Geometry: final body of the model. Coordinates: model frame, mm. A direction names the side the tool comes from. Round coordinates to 2 decimals unless told otherwise and drop trailing zeros. Order: outer loops, then holes, each group sorted by start corner. A loop starts at its lowest first (then second) coordinate and runs counter-clockwise, first axis right, second up. Notation, with made-up numbers: (-30.75, 47.5) -> (-2.75, 47.5) arc R21 cw to (-2.75, 86.5) -> close; hole circle Ø2 at (-6, 42.25). An arc over 180 degrees is marked (long way). Put each result on its own line as item: value.
```python
from build123d import *

# Parameters (mm, degrees)
CROQUIS1_R              = 2.175
SALIENTE_EXTRUIR1_DEPTH = 2
CROQUIS2_W              = 50
CROQUIS2_H              = 25
CORTAR_EXTRUIR1_DEPTH   = 2
REDONDEO1_R             = 5
CORTAR_EXTRUIR2_DEPTH   = 2


with BuildPart() as part:
    # Croquis1 → Saliente-Extruir1 (new body)
    with BuildSketch(Plane(origin=(0, 0, 0), x_dir=(1, 0, 0), z_dir=(0, 1, 0))):
        with BuildLine():
            Line((-59.24665691, 17.931526281), (-59.24665691, -17.931526281))
            ThreePointArc((-59.24665691, -17.931526281), (-56.317724722, -25.002594093), (-49.24665691, -27.931526281))
            Line((-49.24665691, -27.931526281), (-31.500611182, -27.931526281))
            Line((-31.500611182, -27.931526281), (37.914147183, -27.931526281))
            Line((37.914147183, -27.931526281), (59.24665691, -27.931526281))
            Line((59.24665691, -27.931526281), (59.24665691, 17.931526281))
            ThreePointArc((59.24665691, 17.931526281), (56.317724722, 25.002594093), (49.24665691, 27.931526281))
            Line((49.24665691, 27.931526281), (-49.24665691, 27.931526281))
            ThreePointArc((-49.24665691, 27.931526281), (-56.317724722, 25.002594093), (-59.24665691, 17.931526281))
        make_face()
        with Locations((51.3850757, -20.916819625)):
            Circle(CROQUIS1_R, mode=Mode.SUBTRACT)
        with Locations((-41.6149243, -20.916819625)):
            Circle(CROQUIS1_R, mode=Mode.SUBTRACT)
        with Locations((-41.6149243, 20.083180375)):
            Circle(CROQUIS1_R, mode=Mode.SUBTRACT)
        with Locations((51.3850757, 20.083180375)):
            Circle(CROQUIS1_R, mode=Mode.SUBTRACT)
    extrude(amount=SALIENTE_EXTRUIR1_DEPTH)

    # Croquis2 → Cortar-Extruir1 (cut)
    with BuildSketch(Plane(origin=(0, 2, 0), x_dir=(1, 0, 0), z_dir=(0, 1, 0))):
        with Locations((16.3850757, 15.431526281)):
            Rectangle(CROQUIS2_W, CROQUIS2_H)
    extrude(amount=-CORTAR_EXTRUIR1_DEPTH, mode=Mode.SUBTRACT)

    # Redondeo1
    redondeo1_edges = [part.edges().sort_by_distance(p)[0] for p in [
        (41.3850757, 1, -2.931526281),
        (-8.6149243, 1, -2.931526281),
    ]]
    fillet(redondeo1_edges, radius=REDONDEO1_R)

    # Croquis4 → Cortar-Extruir2 (cut)
    with BuildSketch(Plane.XZ):
        with BuildLine():
            Line((29.444521437, 1.568473719), (30.11759836, 1.568473719))
            Line((30.11759836, 1.568473719), (30.11759836, 4.060260578))
            add(Edge.make_bspline(
                [(30.11759836, 4.060260578), (30.148105822, 4.029289813), (30.208706879, 3.967768435), (30.305496315, 3.881954316), (30.405978505, 3.802124559), (30.511147814, 3.729037402), (30.61962941, 3.661651481), (30.732531913, 3.600498497), (30.849036967, 3.544732313), (30.929745062, 3.513567679), (30.970162463, 3.497960898)],
                knots=[0, 0, 0, 0, 0.000130388, 0.000259007, 0.000387777, 0.000515175, 0.000643004, 0.000770695, 0.000900222, 0.001030157, 0.001030157, 0.001030157, 0.001030157], degree=3))
            Line((30.970162463, 3.497960898), (30.970162463, 4.171037821))
            add(Edge.make_bspline(
                [(30.970162463, 4.171037821), (30.925337531, 4.187845247), (30.831522436, 4.223021882), (30.693082905, 4.297844367), (30.548583301, 4.390482153), (30.427195385, 4.481338367), (30.33081837, 4.562116803), (30.263458163, 4.62704999), (30.201045059, 4.693544942), (30.145925041, 4.763747872), (30.096651183, 4.836239432), (30.052992396, 4.910901194), (30.014562629, 4.987969009), (29.994444914, 5.041637327), (29.984385219, 5.068473719)],
                knots=[0, 0, 0, 0, 0.000143475, 0.000300282, 0.000470852, 0.000658192, 0.000754698, 0.000847923, 0.000938715, 0.001028066, 0.00111538, 0.001201478, 0.001287394, 0.001373323, 0.001373323, 0.001373323, 0.001373323], degree=3))
            Line((29.984385219, 5.068473719), (29.444521437, 5.068473719))
            Line((29.444521437, 5.068473719), (29.444521437, 1.568473719))
        make_face()
        with BuildLine():
            Line((0.238227731, 1.568473719), (3.192773185, 1.568473719))
            add(Edge.make_bspline(
                [(3.192773185, 1.568473719), (3.188115357, 1.604788367), (3.178835808, 1.677136155), (3.155068568, 1.784065443), (3.127140852, 1.889748411), (3.092461936, 1.993848095), (3.049680145, 2.095512273), (3.002856429, 2.19669015), (2.94729708, 2.295118176), (2.886860339, 2.394367373), (2.814200344, 2.493443888), (2.729582069, 2.596122101), (2.629633226, 2.701343615), (2.516505876, 2.810695804), (2.389788427, 2.923761308), (2.248649332, 3.040002632), (2.094036264, 3.160927698), (1.984462278, 3.240458026), (1.927858413, 3.281541901)],
                knots=[0, 0, 0, 0, 0.000109782, 0.000218714, 0.000328285, 0.000437662, 0.000547529, 0.000659044, 0.000771901, 0.000886408, 0.001007447, 0.001140123, 0.001285331, 0.001442542, 0.001612054, 0.001794653, 0.001990995, 0.002200805, 0.002200805, 0.002200805, 0.002200805], degree=3))
            add(Edge.make_bspline(
                [(1.927858413, 3.281541901), (1.893424314, 3.306253875), (1.827407407, 3.353631569), (1.734179987, 3.424062611), (1.650525877, 3.490388277), (1.575249679, 3.550647526), (1.510130493, 3.607333231), (1.454212438, 3.658929136), (1.406754234, 3.705389161), (1.358740775, 3.761072032), (1.311519349, 3.826339302), (1.270109393, 3.904031485), (1.242851252, 3.980026103), (1.239730022, 4.031104768), (1.238227731, 4.055689628)],
                knots=[0, 0, 0, 0, 0.000127149, 0.000243769, 0.000350475, 0.000447421, 0.000533008, 0.000609403, 0.000675694, 0.000732085, 0.000829839, 0.000916571, 0.000995853, 0.001069422, 0.001069422, 0.001069422, 0.001069422], degree=3))
            add(Edge.make_bspline(
                [(1.238227731, 4.055689628), (1.239685746, 4.080972097), (1.242541207, 4.130486734), (1.266653205, 4.201654218), (1.305747651, 4.266442593), (1.359509302, 4.323756407), (1.424157163, 4.371621265), (1.498188647, 4.407383572), (1.580621178, 4.428177391), (1.638203662, 4.430771544), (1.667915231, 4.432110082)],
                knots=[0, 0, 0, 0, 7.5688e-05, 0.000148232, 0.000222776, 0.000301178, 0.00038243, 0.000462799, 0.000546343, 0.000635405, 0.000635405, 0.000635405, 0.000635405], degree=3))
            add(Edge.make_bspline(
                [(1.667915231, 4.432110082), (1.698813755, 4.430809048), (1.758278058, 4.428305203), (1.843219818, 4.407324867), (1.918981726, 4.372152378), (1.974530483, 4.331309897), (2.013689853, 4.291349515), (2.040808134, 4.255651482), (2.064355526, 4.214184875), (2.087086891, 4.168265993), (2.105602713, 4.116647385), (2.122002547, 4.059916325), (2.136216017, 3.998020881), (2.14352285, 3.954643819), (2.14731864, 3.932110082)],
                knots=[0, 0, 0, 0, 9.2602e-05, 0.000178213, 0.000260508, 0.00034176, 0.000383446, 0.000428049, 0.000475798, 0.000526305, 0.000581584, 0.000640021, 0.000703423, 0.000771966, 0.000771966, 0.000771966, 0.000771966], degree=3))
            Line((2.14731864, 3.932110082), (3.101864094, 4.006683946))
            add(Edge.make_bspline(
                [(3.101864094, 4.006683946), (3.096994116, 4.039650766), (3.087461692, 4.104179537), (3.067871533, 4.197366087), (3.046962689, 4.285499285), (3.022046312, 4.367704138), (2.994400178, 4.444545826), (2.964137877, 4.515998173), (2.929779719, 4.581157532), (2.881644848, 4.661426522), (2.810389047, 4.751759712), (2.709397011, 4.847015779), (2.592564179, 4.927953002), (2.483825815, 4.984190233), (2.388096824, 5.021729738), (2.308290198, 5.046369437), (2.221990226, 5.067601851), (2.128965037, 5.084403665), (2.029469325, 5.098056751), (1.923011653, 5.106807753), (1.810025667, 5.11265402), (1.732553843, 5.113495947), (1.692773185, 5.113928264)],
                knots=[0, 0, 0, 0, 9.995e-05, 0.000195642, 0.00028556, 0.000371615, 0.000453168, 0.000530478, 0.000604178, 0.000673972, 0.000811075, 0.000947734, 0.001089005, 0.001236077, 0.001313892, 0.001397231, 0.00148646, 0.001580349, 0.001680693, 0.001787626, 0.001900695, 0.002020032, 0.002020032, 0.002020032, 0.002020032], degree=3))
            add(Edge.make_bspline(
                [(1.692773185, 5.113928264), (1.651340679, 5.113397506), (1.570577331, 5.112362914), (1.453036045, 5.107878174), (1.34242277, 5.098420374), (1.23907833, 5.085938383), (1.142821984, 5.069686254), (1.053687032, 5.049772162), (0.971451968, 5.026806196), (0.895920672, 4.999295684), (0.825740946, 4.968820838), (0.760065932, 4.933742155), (0.698346318, 4.894802211), (0.640597303, 4.851866527), (0.586189039, 4.805657255), (0.535953343, 4.755006285), (0.488639596, 4.701098695), (0.446364968, 4.642792682), (0.408254872, 4.582011512), (0.374293308, 4.519431441), (0.347155821, 4.454387488), (0.322843456, 4.388116191), (0.305795233, 4.319440044), (0.292454011, 4.249312564), (0.285675472, 4.177270825), (0.284352217, 4.128617444), (0.283682276, 4.103985082)],
                knots=[0, 0, 0, 0, 0.000124308, 0.000242311, 0.000352782, 0.000457261, 0.000554523, 0.000645501, 0.000731157, 0.000810464, 0.000886471, 0.000960502, 0.001033604, 0.001105196, 0.001176222, 0.001247536, 0.001319026, 0.00139119, 0.001463312, 0.001534167, 0.001604484, 0.00167457, 0.001745713, 0.00181648, 0.001888563, 0.001962482, 0.001962482, 0.001962482, 0.001962482], degree=3))
            add(Edge.make_bspline(
                [(0.283682276, 4.103985082), (0.284146132, 4.077674435), (0.285072563, 4.025125751), (0.295101547, 3.947135962), (0.308857923, 3.869836073), (0.32967374, 3.793603518), (0.356890877, 3.718261121), (0.389668246, 3.643538536), (0.42798763, 3.569681371), (0.472692567, 3.496283619), (0.524647072, 3.422352303), (0.587623536, 3.348689881), (0.658047527, 3.271963933), (0.739230369, 3.194302446), (0.829692238, 3.115067123), (0.930761028, 3.035143861), (1.039488039, 2.951462642), (1.117230695, 2.897900463), (1.157261822, 2.87032031)],
                knots=[0, 0, 0, 0, 7.8886e-05, 0.000157555, 0.000235564, 0.0003143, 0.000394275, 0.000475692, 0.000558919, 0.000643695, 0.000733358, 0.000829659, 0.000934195, 0.001045703, 0.0011665, 0.001294833, 0.001432194, 0.001578003, 0.001578003, 0.001578003, 0.001578003], degree=3))
            add(Edge.make_bspline(
                [(1.157261822, 2.87032031), (1.180969807, 2.854508529), (1.226365633, 2.824232281), (1.29078794, 2.780126058), (1.349326873, 2.74020997), (1.402090118, 2.704045916), (1.448471107, 2.67109448), (1.488355102, 2.641479001), (1.522950215, 2.616823253), (1.561123658, 2.587028109), (1.606631457, 2.549422878), (1.662933813, 2.5008226), (1.723946438, 2.446547502), (1.765107013, 2.407152874), (1.786523185, 2.386655537)],
                knots=[0, 0, 0, 0, 8.549e-05, 0.000163696, 0.00023422, 0.000298049, 0.000355595, 0.000404888, 0.00044708, 0.000483022, 0.000550133, 0.000624164, 0.000706149, 0.000795075, 0.000795075, 0.000795075, 0.000795075], degree=3))
            Line((1.786523185, 2.386655537), (0.238227731, 2.386655537))
            Line((0.238227731, 2.386655537), (0.238227731, 1.568473719))
        make_face()
    extrude(amount=-CORTAR_EXTRUIR2_DEPTH, mode=Mode.SUBTRACT)


solid = part.part
```
1. Draft query along Z for faces 4 (the face through (39.882, 0.986, -4.357)), 5 (the face through (41.385, 1, -18)), 6 (the face through (-40.45, 0.99, -21.92)). Return one class per face: +Z half, -Z half, draft (parallel to the pull), parting line (faces both ways), or undercut.
Ans:
face 4: -Z half
face 5: draft
face 6: undercut
2. Contact query for flat-ended pins moving along their axis: P1, Ø1.2, axis at x = 0.5, y = 0.5, coming from the -Z side; P2, Ø4, axis at x = -41.61, z = -20.08, coming from the +Y side. Output: stop coordinate, or through.
Ans:
P1: z = -2.93
P2: through
3. Set-up query: faces 1 (the face through (4, 1, 27.932)), 2 (the face through (16, 1, -2.932)), 3 (the face through (29.445, 1, 3)). Return all of +Z, -Z, +X, -X, +Y, -Y with unobstructed straight access to the full face (end or side cutting, diameter ignored); none if empty.
Ans:
face 1: +Z, +X, -X, +Y, -Y
face 2: -Z, +Y, -Y
face 3: +Y, -Y
4. Cut plane A-A on x = -41.5. Return loops of the section in (y, z), and give its area (3 significant figures).
Ans:
outline: (0, -27.93) -> (2, -27.93) -> (2, -22.26) -> (0, -22.26) -> close; (0, -17.91) -> (2, -17.91) -> (2, 18.74) -> (0, 18.74) -> close; (0, 23.09) -> (2, 23.09) -> (2, 27.93) -> (0, 27.93) -> close
area: 94.4 mm²
5. Material intervals for probe 1 along Z at (x, y) = (1.5, 1.85); probe 2 along X at (y, z) = (1.8, -12); probe 3 along Z at (x, y) = (29.5, 1.45), sorted ascending.
Ans:
probe 1: -2.93 to 1.57, 2.39 to 2.63, 3.62 to 4.41, 5.11 to 27.93
probe 2: -59.25 to -8.61, 41.39 to 59.25
probe 3: -2.93 to 1.57, 5.07 to 27.93
6. Cut plane C-C on y = 1.6. State how many separate pieces and enclosed holes the cut face has, and give its area (3 significant figures).
Ans:
separate pieces: 1
enclosed holes: 6
area: 5,250 mm²
7. Cut plane B-B on x = 10.5. Return loops of the section in (y, z), and give its area (3 significant figures).
Ans:
outline: (0, -2.93) -> (2, -2.93) -> (2, 27.93) -> (0, 27.93) -> close
area: 61.7 mm²
